Part model, mm, in its own coordinate system. Coordinates: 2 decimals unless noted, no trailing zeros. Loops run counter-clockwise (first coordinate to the right, second up) from the corner with the lowest first, then second, coordinate; pieces in that order, holes last. Notation, with made-up numbers: (4.5, 14) - (23.5, 14) arc R34 cw to (23.5, 44) - close; hole circle Ø7 at (-20, -8). An arc over 180 degrees is marked (long way). Answer as CSV lines item,"result".
from build123d import *

# Parameters (mm, degrees)
SKETCH1_W            = 30.0228
SKETCH1_H            = 12.8016
BOSS_EXTRUDE1_DEPTH  = 7.0104
SKETCH2_W            = 0.508
SKETCH2_H            = 0.3048
BOSS_EXTRUDE2_DEPTH  = 3.9116
LPATTERN1_COUNT      = 4
LPATTERN1_PITCH      = 2.54
LPATTERN1_COUNT_DIR2 = 2
LPATTERN1_PITCH_DIR2 = 10.16
LPATTERN2_COUNT      = 5
LPATTERN2_PITCH      = 2.54
LPATTERN2_COUNT_DIR2 = 2
LPATTERN2_PITCH_DIR2 = 10.16
SKETCH3_R            = 0.5969
CUT_EXTRUDE1_DEPTH   = 0.0254
LPATTERN3_COUNT      = 2
LPATTERN3_PITCH      = 10.16
LPATTERN4_COUNT      = 2
LPATTERN4_PITCH      = 10.16


with BuildPart() as part:
    # Sketch1 → Boss-Extrude1 (new body)
    with BuildSketch(Plane.XY):
        Rectangle(SKETCH1_W, SKETCH1_H)
    extrude(amount=BOSS_EXTRUDE1_DEPTH)

    # Sketch2 → Boss-Extrude2 (add)
    with BuildSketch(Plane(origin=(0, 0, 0), x_dir=(-1, 0, 0), z_dir=(0, 0, -1))):
        with Locations((-1.27, 5.08)):
            Rectangle(SKETCH2_W, SKETCH2_H)
    boss_extrude2 = extrude(amount=BOSS_EXTRUDE2_DEPTH)

    # LPattern1: Boss-Extrude2 4 × 2, 2 skipped
    with Locations(*[(i * LPATTERN1_PITCH, -j * LPATTERN1_PITCH_DIR2, 0) for i in range(LPATTERN1_COUNT) for j in range(LPATTERN1_COUNT_DIR2) if (i, j) not in ((0, 0), (1, 0), (2, 0))]):
        add(boss_extrude2)

    # LPattern2: Boss-Extrude2 5 × 2, 3 skipped
    with Locations(*[(-i * LPATTERN2_PITCH, -j * LPATTERN2_PITCH_DIR2, 0) for i in range(LPATTERN2_COUNT) for j in range(LPATTERN2_COUNT_DIR2) if (i, j) not in ((0, 0), (0, 1), (2, 0), (4, 1))]):
        add(boss_extrude2)

    # Sketch3 → Cut-Extrude1 (cut)
    with BuildSketch(Plane.XY.offset(7.0104)):
        with Locations((3.4925, -4.4069)):
            Circle(SKETCH3_R)
        Polygon((-2.54, 0), (-2.032, 0.508), (2.032, 0.508), (2.54, 0), (2.032, -0.508), (-2.032, -0.508), align=None)
        with BuildLine():
            Line((-2.772210245, 0.127), (-1.821783863, 1.077426382))
            Line((-1.821783863, 1.077426382), (-1.129458257, 5.0038))
            Line((-1.129458257, 5.0038), (-1.734869082, 5.0038))
            ThreePointArc((-1.734869082, 5.0038), (-2.061405188, 4.884950577), (-2.235151421, 4.584013274))
            Line((-2.235151421, 4.584013274), (-3.021043115, 0.127))
            Line((-3.021043115, 0.127), (-2.772210245, 0.127))
        make_face()
        Polygon((0.882304946, 5.0038), (-0.871539898, 5.0038), (-1.047966446, 4.003235323), (0.705878398, 4.003235323), (2.459723242, 4.003235323), (2.63614979, 5.0038), align=None)
        with BuildLine():
            Line((3.24497838, 0.127), (2.772210245, 0.127))
            Line((2.772210245, 0.127), (2.14478817, 0.754422075))
            Line((2.14478817, 0.754422075), (2.89406815, 5.0038))
            Line((2.89406815, 5.0038), (3.499478975, 5.0038))
            ThreePointArc((3.499478975, 5.0038), (3.888629552, 4.822336106), (3.999761313, 4.407586726))
            Line((3.999761313, 4.407586726), (3.24497838, 0.127))
        make_face()
        with BuildLine():
            Line((1.914017295, -5.0038), (1.129458257, -5.0038))
            Line((1.129458257, -5.0038), (1.821783863, -1.077426382))
            Line((1.821783863, -1.077426382), (2.772210245, -0.127))
            Line((2.772210245, -0.127), (3.200191327, -0.127))
            Line((3.200191327, -0.127), (2.414299633, -4.584013274))
            ThreePointArc((2.414299633, -4.584013274), (2.240553401, -4.884950577), (1.914017295, -5.0038))
        make_face()
        with BuildLine():
            Line((-3.065830168, -0.127), (-2.772210245, -0.127))
            Line((-2.772210245, -0.127), (-2.14478817, -0.754422075))
            Line((-2.14478817, -0.754422075), (-2.89406815, -5.0038))
            Line((-2.89406815, -5.0038), (-3.320330762, -5.0038))
            ThreePointArc((-3.320330762, -5.0038), (-3.709481339, -4.822336106), (-3.820613101, -4.407586726))
            Line((-3.820613101, -4.407586726), (-3.065830168, -0.127))
        make_face()
        Polygon((-0.705878398, -4.003235323), (-2.459723242, -4.003235323), (-2.63614979, -5.0038), (-0.882304946, -5.0038), (0.871539898, -5.0038), (1.047966446, -4.003235323), align=None)
    cut_extrude1 = extrude(amount=-CUT_EXTRUDE1_DEPTH, mode=Mode.SUBTRACT)

    # LPattern3: Cut-Extrude1 ×2
    with Locations(*[(i * LPATTERN3_PITCH, 0, 0) for i in range(1, LPATTERN3_COUNT)]):
        add(cut_extrude1, mode=Mode.SUBTRACT)

    # LPattern4: Cut-Extrude1 ×2
    with Locations(*[(-i * LPATTERN4_PITCH, 0, 0) for i in range(1, LPATTERN4_COUNT)]):
        add(cut_extrude1, mode=Mode.SUBTRACT)


solid = part.part
Q1. Wall check: L1, parallel to Z at x = 9, y = -2.5. Give the ranges that are in metal, low to high.
Results:
L1,"z = 0 to 7.01"
Q2. Saw through at D-D (x = 5). Give the cut face in (y, z), then the cut area to 3 significant figures.
Results:
outline,"(-6.4, 0) - (6.4, 0) - (6.4, 7.01) - (-6.4, 7.01) - close"
area,"89.7 mm^2"
Q3. Saw through at C-C (y = -3). Give the cut face in (x, z) (3 decimals), then the cut area to 3 significant figures.
Results:
outline,"(-15.011, 0) - (15.011, 0) - (15.011, 7.01) - (12.854, 7.01) - (12.854, 6.985) - (11.643, 6.985) - (11.643, 7.01) - (7.619, 7.01) - (7.619, 6.985) - (6.588, 6.985) - (6.588, 7.01) - (2.694, 7.01) - (2.694, 6.985) - (1.483, 6.985) - (1.483, 7.01) - (-2.541, 7.01) - (-2.541, 6.985) - (-3.572, 6.985) - (-3.572, 7.01) - (-7.466, 7.01) - (-7.466, 6.985) - (-8.677, 6.985) - (-8.677, 7.01) - (-12.701, 7.01) - (-12.701, 6.985) - (-13.732, 6.985) - (-13.732, 7.01) - (-15.011, 7.01) - close"
area,"210 mm^2"
Q4. Saw through at A-A (x = -10.5). Give the cut face in (y, z) (3 decimals), then the cut area to 3 significant figures.
Results:
outline,"(-6.401, 0) - (6.401, 0) - (6.401, 7.01) - (5.004, 7.01) - (5.004, 6.985) - (4.003, 6.985) - (4.003, 7.01) - (0.508, 7.01) - (0.508, 6.985) - (-0.508, 6.985) - (-0.508, 7.01) - (-4.003, 7.01) - (-4.003, 6.985) - (-5.004, 6.985) - (-5.004, 7.01) - (-6.401, 7.01) - close"
area,"89.7 mm^2"
Q5. Two-plate mould, pull along Y, no slides. Class faces 1 (the face through (-10, 0, 6.985)), 2 (the face through (15.011, 0, 3)), 3 (the face through (12, -3, 6.985)), 4 (the face through (0, -6.401, 3)): released by +Y, released by -Y, zero draft, split by the parting line, or undercut.
Results:
face 1,"undercut"
face 2,"zero draft"
face 3,"undercut"
face 4,"released by -Y"
Q6. Saw through at B-B (z = -0.5). Count the separate pieces of the cut face and the enclosed holes in it, then the cut area to 3 significant figures.
Results:
separate pieces,"12"
enclosed holes,"0"
area,"1.86 mm^2"
Q7. Flat gauge pins, fed straight in: pin 1 (0.6 mm diameter, centred on x = -6.5, z = -2.5, fed in from -Y); pin 2 (0.8 mm diameter, centred on x = -13, y = -3.5, fed in from +Z); pin 3 (4 mm diameter, centred on x = 8.5, y = -1.5, fed in from -Z). Where does each tip first touch, or does it go through?
Results:
pin 1,"stops at y = -5.23"
pin 2,"stops at z = 7.01"
pin 3,"stops at z = 0"
